```python
from build123d import *

# Parameters (mm, degrees)
F4_T = 10


with BuildPart() as f3:
    # F0 (on Top) → F3 section 0
    with BuildSketch(Plane.XY):
        Polygon((0, 505), (0, 0), (918, 0), (917.9733111534, 497.9999992848), align=None)
    # F2 (on offset) → F3 section 1
    with BuildSketch(Plane.XY.offset(2090)):
        Polygon((0, 509), (0, 0), (920, 0), (929.6877679676, 484.9032348333), align=None)
    loft()

    # F4
    f4_openings = [f3.faces().sort_by_distance(p)[0] for p in [
        (459.500181, 0, 1045.379035),
    ]]
    offset(amount=F4_T, openings=f4_openings, kind=Kind.INTERSECTION)


solid = f3.part
```
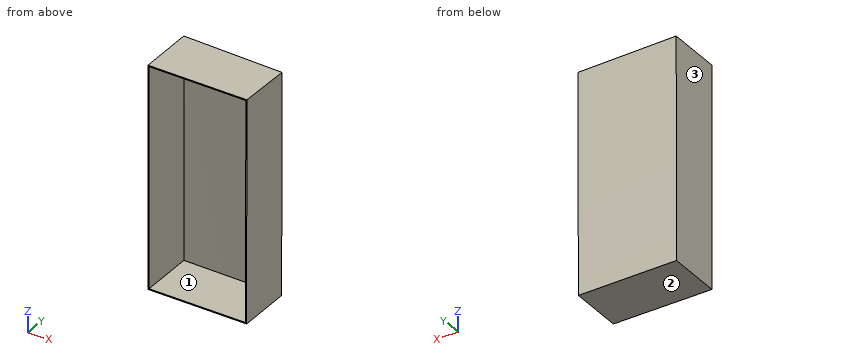
Read the model definition and answer for the solid it produces. Units are mm, in the model's axes. Face numbers are marked on the shaded views. Round coordinates to 2 decimals unless told otherwise and drop trailing zeros. Use CSV: the item, a comma, the result in double quotes.
Q1. Each of these flat-tipped pins is pushed along its axis until it touches: pin 1 Ø8 at (x, z) = (749.5, 987.5) entering from +Y; pin 2 Ø1 at (y, z) = (301, 424) entering from +X. Where does it stop, or does it pass through?
Values:
pin 1,"stops at y = 504.72"
pin 2,"stops at x = 929.59"
Q2. Straight lines are drawn through the part: line 1 along Z through (x, y) = (350, 127.5); line 2 along X through (y, z) = (23, 306); line 3 along X through (y, z) = (128, 1326). For each, find the intervals that lie inside material, in ascending order.
Values:
line 1,"z = -10 to 0, 2090 to 2100"
line 2,"x = -10 to 0, 918.36 to 928.36"
line 3,"x = -10 to 0, 920.87 to 930.87"
Q3. Determine the mould class of the marked faces 1, 2 and 3 for opening direction X: +X half, -X half, draft (parallel to the pull), parting line (faces both ways), or undercut.
Values:
face 1,"undercut"
face 2,"draft"
face 3,"-X half"
